Part model, mm, in its own coordinate system. Face numbers are marked on the shaded views. A direction names the side the tool comes from. Give positions to 0.01 mm unless a question says otherwise; leave off trailing zeros. Order: outer loops, then holes, each group sorted by start corner. A loop starts at its lowest first (then second) coordinate and runs counter-clockwise, first axis right, second up. Notation, with made-up numbers: (89.5, 8) -> (134.5, 8) arc R28 ccw to (134.5, 43) -> close; hole circle Ø10 at (16, 14). An arc over 180 degrees is marked (long way). Write item = value, one per line. Start each with the question number.
Item 1: Pull direction X, two halves, no side cores. Call the marked faces 1, 2 and 3: +X half, -X half, draft (parallel to the pull), parting line (faces both ways), or undercut.
Item 2: Band-saw the part on A-A on y = -19.5. Write the cut outline in (x, z).
Item 3: Band-saw the part on B-B on x = 0. Write the cut outline in (y, z), plus the area to 3 significant figures.
Item 4: Drill centre lines: line 1 along Z through (x, y) = (4, -8.5); line 2 along X through (y, z) = (-10.5, -25); line 3 along Y through (x, z) = (11, 17). Where is each one in solid material? Low to high.
Item 5: Flat gauge pins, fed straight in: P1, Ø5, axis at y = -7.5, z = 18, coming from the +X side; P2, Ø3, axis at y = -5, z = 13, coming from the -X side; P3, Ø10, axis at x = 6, y = -12, coming from the -Z side. Where does each tip first touch, or does it go through?
Item 6: Band-saw the part on D-D on y = -27. Write the cut outline in (x, z), plus the area to 3 significant figures.
Item 7: Band-saw the part on C-C on z = 0. Write the cut outline in (x, y), plus the area to 3 significant figures.
Item 8: Tool access for the marked faces 4 and 5: list every direction of +Z, -Z, +X, -X, +Y, -Y with a clear straight run to the whole face (end or side of a thin tool).
```python
from build123d import *

# Parameters (mm, degrees)
F0_R        = 27
F1_DEPTH    = 5.08
F3_DEPTH    = 25.4
F4_T1_DEPTH = 33.0899649141
F4_T3_DEPTH = 33.0899649141
F4_T5_DEPTH = 33.0899649141


# Not quite as in the source:
# - a fillet or chamfer that OpenCascade refuses, or shapes differently, is made with other operations: its cross-section is extruded or revolved along the edge and cut away or added


with BuildPart() as f1:
    # F0 (on Front) → F1 (new body)
    with BuildSketch(Plane.XZ):
        Circle(F0_R)
    extrude(amount=F1_DEPTH)

    # F2 (on face) → F3 (join)
    with BuildSketch(Plane.XZ.offset(5.08)):
        with BuildLine():
            ThreePointArc((-25.4641942221, 8.9763473985), (-25.4782526607, 8.9363662278), (-25.4922483252, 8.8963630393))
            Line((-25.4922483252, 8.8963630393), (-22.90776578, 7.4042113462))
            Line((-22.90776578, 7.4042113462), (-17.90776578, 16.064465384))
            Line((-17.90776578, 16.064465384), (-20.5058419913, 17.564465384))
            Line((-20.5058419913, 17.564465384), (-25.4641942221, 8.9763473985))
        make_face()
        with BuildLine():
            Line((22.8661180108, 7.4763473985), (25.4641942221, 8.9763473985))
            Line((25.4641942221, 8.9763473985), (20.5058419913, 17.564465384))
            ThreePointArc((20.5058419913, 17.564465384), (20.4782465011, 17.5966309343), (20.4506005559, 17.6287531295))
            Line((20.4506005559, 17.6287531295), (17.8661180108, 16.1366014363))
            Line((17.8661180108, 16.1366014363), (22.8661180108, 7.4763473985))
        make_face()
        with BuildLine():
            Line((-4.9583522308, -23.5408127825), (-4.9583522308, -26.5408127825))
            Line((-4.9583522308, -26.5408127825), (4.9583522308, -26.5408127825))
            ThreePointArc((4.9583522308, -26.5408127825), (5.0000061596, -26.5329971621), (5.0416477692, -26.5251161689))
            Line((5.0416477692, -26.5251161689), (5.0416477692, -23.5408127825))
            Line((5.0416477692, -23.5408127825), (-4.9583522308, -23.5408127825))
        make_face()
    extrude(amount=F3_DEPTH)

    # F4: fillet of radius 5.08 on 3 edges, made by hand

    # F4_s2 → F4_t1 (cut)
    with BuildSketch(Plane(origin=(8.2724912285, 0, 14.328375113), x_dir=(0, 1, 0), z_dir=(-0.5, 0, -0.8660254038))):
        with BuildLine():
            ThreePointArc((-25.8453479095, -26.5408127825), (-28.6057826579, -25.7253643416), (-30.48, -23.5408127825))
            Line((-30.48, -23.5408127825), (-30.48, -26.5408127825))
            Line((-30.48, -26.5408127825), (-25.8453479095, -26.5408127825))
        make_face()
    extrude(amount=F4_T1_DEPTH, mode=Mode.SUBTRACT)

    # F4_s4 → F4_t3 (cut)
    with BuildSketch(Plane.YZ.offset(-16.544982457)):
        with BuildLine():
            ThreePointArc((-25.8453479095, -26.5408127825), (-28.6057826579, -25.7253643416), (-30.48, -23.5408127825))
            Line((-30.48, -23.5408127825), (-30.48, -26.5408127825))
            Line((-30.48, -26.5408127825), (-25.8453479095, -26.5408127825))
        make_face()
    extrude(amount=F4_T3_DEPTH, mode=Mode.SUBTRACT)

    # F4_s6 → F4_t5 (cut)
    with BuildSketch(Plane(origin=(8.2724912285, 0, -14.328375113), x_dir=(0, 1, 0), z_dir=(-0.5, 0, 0.8660254038))):
        with BuildLine():
            ThreePointArc((-25.8453479095, -26.5408127825), (-28.6057826579, -25.7253643416), (-30.48, -23.5408127825))
            Line((-30.48, -23.5408127825), (-30.48, -26.5408127825))
            Line((-30.48, -26.5408127825), (-25.8453479095, -26.5408127825))
        make_face()
    extrude(amount=F4_T5_DEPTH, mode=Mode.SUBTRACT)


solid = f1.part
```
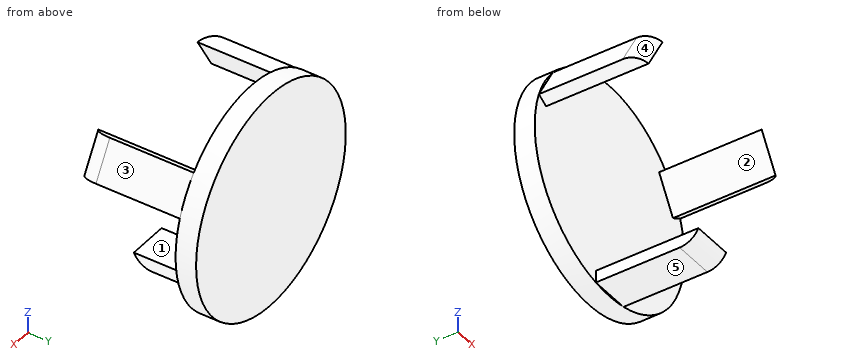
Values found:
q1.face_1 = draft
q1.face_2 = undercut
q1.face_3 = +X half
q2.outline = (-25.49, 8.9) -> (-22.91, 7.4) -> (-17.91, 16.06) -> (-20.51, 17.56) -> (-25.46, 8.98) arc R27 ccw to start; (-4.96, -26.54) -> (4.96, -26.54) arc R27 ccw to (5.04, -26.53) -> (5.04, -23.54) -> (-4.96, -23.54) -> close; (17.87, 16.14) -> (22.87, 7.48) -> (25.46, 8.98) -> (20.51, 17.56) arc R27 ccw to (20.45, 17.63) -> close
q3.outline = (-30.48, -23.54) arc R5.08 ccw to (-25.85, -26.54) -> (-5.08, -26.54) -> (-5.08, -27) -> (0, -27) -> (0, 27) -> (-5.08, 27) -> (-5.08, -23.54) -> close
q3.area = 347 mm^2
q4.line_1 = -26.54 to -23.54
q4.line_2 = -4.96 to 5.04
q4.line_3 = -5.08 to 0
q5.P1 = 21.7
q5.P2 = -24.43
q5.P3 = -26.54
q6.outline = (-25.39, 8.84) -> (-22.91, 7.4) -> (-17.91, 16.06) -> (-20.39, 17.5) -> close; (-4.96, -26.41) -> (5.04, -26.41) -> (5.04, -23.54) -> (-4.96, -23.54) -> close; (17.87, 16.14) -> (22.87, 7.48) -> (25.35, 8.91) -> (20.35, 17.57) -> close
q6.area = 86.0 mm^2
q7.outline = (-27, -5.08) -> (27, -5.08) -> (27, 0) -> (-27, 0) -> close
q7.area = 274 mm^2
q8.face_4 = +Z, -X, -Y
q8.face_5 = -Z, +X, -X, -Y
